Geometry: final body of the model. Coordinates: model frame, mm. A direction names the side the tool comes from. Give positions to 0.01 mm unless a question says otherwise; leave off trailing zeros. Write each loop counter-clockwise with the first axis right and the second up, starting at its lowest first coordinate (ties: lowest second). Pieces come first, ordered by that corner, then holes. Notation, with made-up numbers: (3.25, 26) -> (16.25, 26) arc R20 cw to (16.25, 42) -> close; hole circle Ø11 at (57, -32.75). An arc over 180 degrees is marked (long way). Answer as a JSON object with one key per item and string values.
from build123d import *

# Parameters (mm, degrees)
SKETCH1_R           = 1.5
BOSS_EXTRUDE1_DEPTH = 2
SKETCH2_W           = 7
SKETCH2_H           = 6
BOSS_EXTRUDE2_DEPTH = 5
SKETCH3_R           = 1.5
BOSS_EXTRUDE3_DEPTH = 2
FILLET1_R           = 2


with BuildPart() as part:
    # Sketch1 → Boss-Extrude1 (new body)
    with BuildSketch(Plane(origin=(0, 0, 0), x_dir=(0, 0, -1), z_dir=(1, 0, 0))):
        with BuildLine():
            Line((-11.5, 3), (11.5, 3))
            ThreePointArc((11.5, 3), (14.5, 0), (11.5, -3))
            Line((11.5, -3), (-11.5, -3))
            ThreePointArc((-11.5, -3), (-14.5, 0), (-11.5, 3))
        make_face()
        with Locations((-11.5, 0)):
            Circle(SKETCH1_R, mode=Mode.SUBTRACT)
        with Locations((11.5, 0)):
            Circle(SKETCH1_R, mode=Mode.SUBTRACT)
    extrude(amount=BOSS_EXTRUDE1_DEPTH)

    # Sketch2 → Boss-Extrude2 (add)
    with BuildSketch(Plane(origin=(2, 0, 0), x_dir=(0, 0, -1), z_dir=(1, 0, 0))):
        Rectangle(SKETCH2_W, SKETCH2_H)
    extrude(amount=BOSS_EXTRUDE2_DEPTH)

    # Sketch3 → Boss-Extrude3 (add)
    with BuildSketch(Plane(origin=(7, 0, 0), x_dir=(0, 0, -1), z_dir=(1, 0, 0))):
        with BuildLine():
            Line((11.5, 3), (-11.5, 3))
            ThreePointArc((-11.5, 3), (-14.5, 0), (-11.5, -3))
            Line((-11.5, -3), (11.5, -3))
            ThreePointArc((11.5, -3), (14.5, 0), (11.5, 3))
        make_face()
        with Locations((11.5, 0)):
            Circle(SKETCH3_R, mode=Mode.SUBTRACT)
        with Locations((-11.5, 0)):
            Circle(SKETCH3_R, mode=Mode.SUBTRACT)
    extrude(amount=BOSS_EXTRUDE3_DEPTH)

    # Fillet1
    fillet1_edges = [part.edges().sort_by_distance(p)[0] for p in [
        (2, 0, -3.5),
        (2, 0, 3.5),
        (7, 0, -3.5),
        (7, 0, 3.5),
    ]]
    fillet(fillet1_edges, radius=FILLET1_R)


solid = part.part
Q1. Material intervals for L1, parallel to X at y = 2.55, z = 12.75; L2, parallel to Z at x = 8.25, y = 1.2; L3, parallel to Y at x = 1.65, z = 11.5, sorted ascending. Write a range as from..to.
Values:
{"L1": "0..2, 7..9", "L2": "-14.25..-12.4, -10.6..10.6, 12.4..14.25", "L3": "-3..-1.5, 1.5..3"}
Q2. First-contact query: P1, Ø1, axis at y = -2, z = -6, coming from the -X side; P2, Ø2.5, axis at y = 0, z = -11.5, coming from the -X side. Flat tips, straight axial feed; report the tip coordinate or a pass-through.
Values:
{"P1": "x = 0", "P2": "through"}
Q3. Cut plane C-C (x = 4.5). Return the cut outline in (y, z).
Values:
{"outline": "(-3, -3.5) -> (3, -3.5) -> (3, 3.5) -> (-3, 3.5) -> close"}
Q4. Set-up query: faces 4 (the flat face through (4.5, 0, 3.5)), 5 (the cylindrical face through (2.6, 0.04, -4.07)), 6 (the cylindrical face through (1, 0, -10)). Return all of +Z, -Z, +X, -X, +Y, -Y with unobstructed straight access to the full face (end or side cutting, diameter ignored); none if empty.
Values:
{"face 4": "+Z, +Y, -Y", "face 5": "-Z, +Y, -Y", "face 6": "+X, -X"}
Q5. Cut plane A-A (z = 7.75). Return the cut outline in (x, y).
Values:
{"outline": "(0, -3) -> (2, -3) -> (2, 3) -> (0, 3) -> close; (7, -3) -> (9, -3) -> (9, 3) -> (7, 3) -> close"}
Q6. Cut plane D-D (y = -1.9). Return the cut outline in (x, z).
Values:
{"outline": "(0, -13.82) -> (2, -13.82) -> (2, -5.5) arc R2 cw to (4, -3.5) -> (5, -3.5) arc R2 cw to (7, -5.5) -> (7, -13.82) -> (9, -13.82) -> (9, 13.82) -> (7, 13.82) -> (7, 5.5) arc R2 cw to (5, 3.5) -> (4, 3.5) arc R2 cw to (2, 5.5) -> (2, 13.82) -> (0, 13.82) -> close"}
Q7. Cut plane B-B (y = 0). State how many separate pieces and enclosed holes the cut face has, and give its area (3 significant figures).
Values:
{"separate pieces": "5", "enclosed holes": "0", "area": "130 mm²"}
Q8. Mould query, pull axis X, two halves, no side actions, for faces 1 (the cylindrical face through (8, 0.1, 14.5)), 2 (the flat face through (0, 0, 0)), 3 (the cylindrical face through (6.43, 0.04, 4.1)). Classes: pulls with the +X half, pulls with the -X half, needs draft (parallel to the pull), parting line crosses it, or undercut.
Values:
{"face 1": "needs draft", "face 2": "pulls with the -X half", "face 3": "undercut"}
